Autodesk Inventor part; units mm, degrees
ref_plane "YZ Plane" through (0, 0, 0) normal (1, 0, 0) x (0, 1, 0)
ref_plane "XZ Plane" through (0, 0, 0) normal (0, 1, 0) x (-1, 0, 0)
ref_plane "XY Plane" through (0, 0, 0) normal (0, 0, 1) x (1, 0, 0)
sketch "Skizze1" plane through (0, 0, 0) normal (0, 0, 1) x (1, 0, 0)
  line L0 (0, 5.6) -> (0, -5.6) construction
  line L1 (-9.1, 0) -> (26.6, 0) construction
  circle A0 centre (0, 0) radius 2
  circle A1 centre (9.5, 0) radius 1
  circle A2 centre (16, 0) radius 1
  circle A3 centre (19, 0) radius 1
  arc A4 (19.1974, -2.4922) -> (19.1974, 2.4922) centre (19, 0) ccw
  arc A5 (0.3158, 3.9875) -> (0.3158, -3.9875) centre (0, 0) ccw
  line L2 (0.3158, 3.9875) -> (19.1974, 2.4922)
  line L3 (0.3158, -3.9875) -> (19.1974, -2.4922)
  circle A6 centre (6, 0) radius 1
  circle A7 centre (12.8, 0) radius 1
  circle A8 centre (0, 0) radius 4
  point P0 (0.5263, 3.9652)
  point P1 (0.6579, -1.8887)
  point P2 (0.6579, 1.8887)
  dimension "d0" = 9.5
  dimension "d1" = 16
  dimension "d2" = 19
  dimension "d3" = 5
  dimension "d4" = 2
  dimension "d5" = 4
  dimension "d6" = 8
  dimension "d16" = 6
  dimension "d17" = 12.8
extrude "Extrusion1" add sketch "Skizze1" along normal blind 2
extrude "Extrusion2" add sketch "Skizze1" along normal blind 3 contours A5 A8
properties part number "Servo-Arm-20mm"
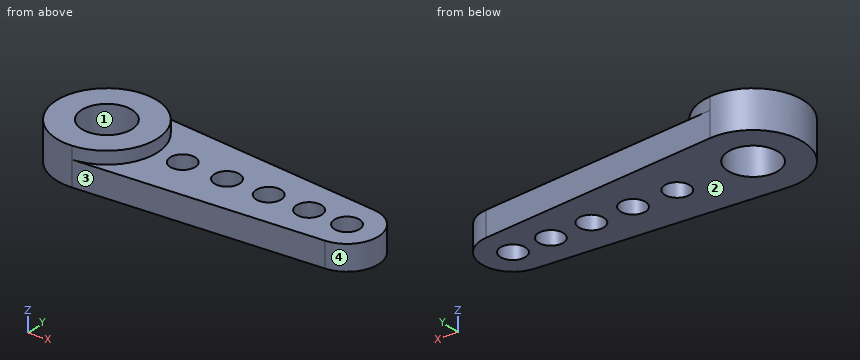
Geometry check sheet. Reference: the model listing, model coordinates, mm. Face numbers are marked on the shaded views. Coordinates: 2 decimals unless noted, no trailing zeros. Order: outer loops, then holes, each group sorted by start corner. A loop starts at its lowest first (then second) coordinate and runs counter-clockwise, first axis right, second up. Notation, with made-up numbers: M -39,16 L -23,16 A21 cw -23,20 Z; hole C -25,64 d7. An arc over 180 degrees is marked long. Answer as a JSON object with one key per item and string values.
Q1. Scan lines: line 1 (Z direction, x = 9.5, y = -2.75); line 2 (X direction, y = -0.5, z = 2.4); line 3 (X direction, y = -1.25, z = 2.2). Record each from-to range of solid material in increasing order.
Results are:
{"line 1": "z = 0 to 2", "line 2": "x = -3.97 to -1.94, 1.94 to 3.97", "line 3": "x = -3.8 to -1.56, 1.56 to 3.8"}
Q2. Release check for a two-part mould opening along Y. For the marked faces 1, 2, 3 and 4 record: released by +Y, released by -Y, zero draft, split by the parting line, or undercut.
Results are:
{"face 1": "undercut", "face 2": "zero draft", "face 3": "released by -Y", "face 4": "split by the parting line"}
Q3. Cross-section at C-C on y = 0. Give the number of separate pieces and of enclosed holes in the cut face, and give its area (3 significant figures).
Results are:
{"separate pieces": "7", "enclosed holes": "0", "area": "27.0 mm²"}
Q4. Cross-section at D-D on y = 1.25. Record the cut outline in (x, z).
Results are:
{"outline": "M -3.8,0 L -1.56,0 L -1.56,3 L -3.8,3 Z; M 1.56,0 L 21.17,0 L 21.17,2 L 3.8,2 L 3.8,3 L 1.56,3 Z"}
Q5. Cross-section at A-A on z = 1.5. Record the cut outline in (x, y), and give its area (3 significant figures).
Results are:
{"outline": "M 0.32,-3.99 L 19.2,-2.49 A2.5 ccw 19.2,2.49 L 0.32,3.99 A4 ccw long Z; hole C 0,0 d4; hole C 6,0 d2; hole C 9.5,0 d2; hole C 12.8,0 d2; hole C 16,0 d2; hole C 19,0 d2", "area": "131 mm²"}
Q6. Depth check by flat-ended pin: pin 1 Ø1.2 at (x, y) = (6, 0) entering from -Z; pin 2 Ø2.5 at (x, y) = (19, 0) entering from +Z; pin 3 Ø1 at (x, z) = (10.5, 1.5) entering from -Y. Enter the tip coordinate at first touch or a pass-through.
Results are:
{"pin 1": "passes through", "pin 2": "stops at z = 2", "pin 3": "stops at y = -3.22"}
Q7. Cross-section at B-B on x = 0. Record the cut outline in (y, z), and give its area (3 significant figures).
Results are:
{"outline": "M -4,0 L -2,0 L -2,3 L -4,3 Z; M 2,0 L 4,0 L 4,3 L 2,3 Z", "area": "12.0 mm²"}
